The model under review builds one solid part; all positions refer to its coordinate system, in mm. Coordinates: 2 decimals unless noted, no trailing zeros. Loops run counter-clockwise (first coordinate to the right, second up) from the corner with the lowest first, then second, coordinate; pieces in that order, holes last. Notation, with made-up numbers: M 5,-30.5 L 18,-30.5 A15 ccw 18,-5.5 Z; hole C -34,86 d1. An arc over 180 degrees is marked long. Use CSV: the item, a comma, the result in double quotes. Start each with the question number.
1. Add section D-D, the plane z = -3.25. Write out the cut boundary in (x, y).
2. Draft analysis for pull direction X (two halves, no side actions). For faces 1 (the conical face through (0.41, -1.87, 6.33)), 2 (the flat face through (-3, -10, -11)), 3 (the cylindrical face through (-14.985, 0.66, 10.493)), 4 (the conical face through (0.41, 1.87, -6.33)), state which applies: +X half, -X half, draft (parallel to the pull), parting line (faces both ways), or undercut.
3. Clearance check with flat-ended pins moving along their axes: P1, Ø8, axis at x = 10, z = 2, coming from the +Y side; P2, Ø3, axis at x = 5.5, z = 3.5, coming from the +Y side (3 decimals); P3, Ø3, axis at x = 4, y = -4.5, coming from the +Z side; P4, Ø2, axis at x = -6, y = -1, coming from the -Z side. State where each tip first meets the part, or that it passes through.
4. Add section A-A, the plane y = 0. Write out the cut boundary in (x, z), then the cut area to 3 significant figures.
5. For L1, parallel to Z at x = -1.5, y = -10.5; L2, parallel to Z at x = 7.5, y = 11.25; L3, parallel to Y at x = 0, z = 2, list the stretches that pass through material, from the lowest coordinate up.
6. Add section C-C, the plane z = 3. Write out the cut boundary in (x, y).
from build123d import *

# Parameters (mm, degrees)
F2_DEPTH       = 1
F3_DEPTH       = 1
F5_D           = 3
F5_DEPTH       = 11
F5_CSINK_D     = 20
F5_CSINK_ANGLE = 120
F5_TIP         = 0.9012909285
F7_D           = 3
F7_DEPTH       = 11
F7_CSINK_D     = 20
F7_CSINK_ANGLE = 120
F7_TIP         = 0.9012909285


with BuildPart() as f1:
    # F0 (on Front) → F1 (revolve)
    with BuildSketch(Plane.XZ):
        with BuildLine():
            ThreePointArc((15, -10), (5, 0), (15, 10))
            Line((15, 10), (0, 10))
            Line((0, 10), (0, -10))
            Line((0, -10), (15, -10))
        make_face()
    revolve(axis=Axis((0, 0, 0), (0, 0, 1)))

    # F2 (add): a face of the model
    f2_faces = [f1.faces().sort_by_distance(p)[0] for p in [
        (0, 0, 10),
    ]]
    extrude(f2_faces, amount=F2_DEPTH)

    # F3 (add): a face of the model
    f3_faces = [f1.faces().sort_by_distance(p)[0] for p in [
        (0, 0, -10),
    ]]
    extrude(f3_faces, amount=F3_DEPTH)

    # F5
    with Locations(Plane.XY.offset(11)):
        with Locations((0, 0)):
            CounterSinkHole(F5_D / 2, F5_CSINK_D / 2, depth=F5_DEPTH, counter_sink_angle=F5_CSINK_ANGLE)
            with Locations((0, 0, -(F5_DEPTH + F5_TIP / 2))):  # 118° drill point
                Cone(0, F5_D / 2, F5_TIP, mode=Mode.SUBTRACT)

    # F7
    with Locations(Plane(origin=(0, 0, -11), x_dir=(1, 0, 0), z_dir=(0, 0, -1))):
        with Locations((0, 0)):
            CounterSinkHole(F7_D / 2, F7_CSINK_D / 2, depth=F7_DEPTH, counter_sink_angle=F7_CSINK_ANGLE)
            with Locations((0, 0, -(F7_DEPTH + F7_TIP / 2))):  # 118° drill point
                Cone(0, F7_D / 2, F7_TIP, mode=Mode.SUBTRACT)


solid = f1.part
Computed:
1,outline,"C 0,0 d11.09; hole C 0,0 d3"
2,face 1,"undercut"
2,face 2,"draft"
2,face 3,"parting line"
2,face 4,"undercut"
3,P1,"passes through"
3,P2,"stops at y = 4.215"
3,P3,"stops at z = 9.57"
3,P4,"stops at z = -9.32"
4,outline,"M -15,-11 L -10,-11 L -1.5,-6.09 L -1.5,6.09 L -10,11 L -15,11 L -15,10 A10 cw -15,-10 Z; M 1.5,-6.09 L 10,-11 L 15,-11 L 15,-10 A10 cw 15,10 L 15,11 L 10,11 L 1.5,6.09 Z"
4,area,"196 mm^2"
5,L1,"z = -11 to -8.98, 8.98 to 11"
5,L2,"z = -11 to -9.89, 9.89 to 11"
5,L3,"y = -5.2 to -1.5, 1.5 to 5.2"
6,outline,"C 0,0 d10.92; hole C 0,0 d3"
